Can you work these out from the model? Positions are in its coordinate system, mm. Face numbers are marked on the shaded views. A direction names the side the tool comes from. Round coordinates to 2 decimals unless told otherwise and drop trailing zeros. Order: outer loops, then holes, each group sorted by start corner. A loop starts at its lowest first (then second) coordinate and runs counter-clockwise, first axis right, second up. Notation, with made-up numbers: (76, 47) -> (84, 47) arc R14 cw to (84, 57) -> close; hole circle Ø10 at (20, -23.5). An arc over 180 degrees is marked (long way). One line per item, written item: value.
```python
from build123d import *

# Parameters (mm, degrees)
SKETCH1_R                = 6.35
BOSS_EXTRUDE1_DEPTH      = 19.05
SKETCH2_R                = 19.05
BOSS_EXTRUDE2_DEPTH      = 25.4
SKETCH3_R                = 25.4
BOSS_EXTRUDE3_DEPTH      = 38.1
SKETCH4_R                = 19.05
BOSS_EXTRUDE4_DEPTH      = 25.4
SKETCH6_R                = 6.35
BOSS_EXTRUDE5_DEPTH      = 28.194
SKETCH8_R                = 12.7
SKETCH8_R_2              = 9.525
BOSS_EXTRUDE7_DEPTH      = 38.1
BOSS_EXTRUDE8_DEPTH      = 1.5875
BOSS_EXTRUDE8_DEPTH_BACK = 1.5875
FILLET1_R                = 2.54
FILLET3_R                = 1.27
CUT_EXTRUDE1_REACH       = 145.927
SKETCH10_R               = 0.492787201


with BuildPart() as part:
    # Sketch1 → Boss-Extrude1 (new body)
    with BuildSketch(Plane(origin=(0, 0, 0), x_dir=(1, 0, 0), z_dir=(0, 1, 0))):
        with Locations(Location((0, 0, 0), (0, 0, 90))):
            Circle(SKETCH1_R)
    extrude(amount=BOSS_EXTRUDE1_DEPTH)

    # Sketch2 → Boss-Extrude2 (add)
    with BuildSketch(Plane(origin=(0, 19.05, 0), x_dir=(1, 0, 0), z_dir=(0, 1, 0))):
        with Locations(Location((0, 0, 0), (0, 0, 270))):
            Circle(SKETCH2_R)
    extrude(amount=BOSS_EXTRUDE2_DEPTH)

    # Sketch3 → Boss-Extrude3 (add)
    with BuildSketch(Plane(origin=(0, 44.45, 0), x_dir=(1, 0, 0), z_dir=(0, 1, 0))):
        with Locations(Location((0, 0, 0), (0, 0, 90))):
            Circle(SKETCH3_R)
    extrude(amount=BOSS_EXTRUDE3_DEPTH)

    # Sketch4 → Boss-Extrude4 (add)
    with BuildSketch(Plane(origin=(0, 82.55, 0), x_dir=(1, 0, 0), z_dir=(0, 1, 0))):
        with Locations(Location((0, 0, 0), (0, 0, 270))):
            Circle(SKETCH4_R)
    extrude(amount=BOSS_EXTRUDE4_DEPTH)

    # Sketch6 → Boss-Extrude5 (add)
    with BuildSketch(Plane(origin=(0, 107.95, 0), x_dir=(1, 0, 0), z_dir=(0, 1, 0))):
        with Locations(Location((0, 0, 0), (0, 0, 90))):
            Circle(SKETCH6_R)
    extrude(amount=BOSS_EXTRUDE5_DEPTH)

    # Sketch8 → Boss-Extrude7 (add)
    with BuildSketch(Plane(origin=(0, 0, 0), x_dir=(0, 0, -1), z_dir=(1, 0, 0))):
        with Locations(Location((0, 62.6872, 0), (0, 0, 180))):
            Circle(SKETCH8_R)
        with Locations(Location((0, 62.6872, 0), (0, 0, 180))):
            Circle(SKETCH8_R_2, mode=Mode.SUBTRACT)
    extrude(amount=BOSS_EXTRUDE7_DEPTH)

    # Sketch9 → Boss-Extrude8 (add, two sides: drawn at the far end of the back side and taken through both)
    with BuildSketch(Plane.XY.offset(-BOSS_EXTRUDE8_DEPTH_BACK)):
        with BuildLine():
            Line((8.114515419, 125.073963283), (6.806070155, 123.814961738))
            Line((6.806070155, 123.814961738), (-6.937623928, 123.814961738))
            ThreePointArc((-6.937623928, 123.814961738), (-7.582023221, 123.584458747), (-7.934028883, 122.997539593))
            Line((-7.934028883, 122.997539593), (-10.230756182, 111.473241157))
            ThreePointArc((-10.230756182, 111.473241157), (-10.582761844, 110.886322003), (-11.227161138, 110.655819012))
            Line((-11.227161138, 110.655819012), (-11.332644522, 110.655819012))
            ThreePointArc((-11.332644522, 110.655819012), (-12.11814153, 111.027419718), (-12.329049477, 111.870396866))
            Line((-12.329049477, 111.870396866), (-9.688493735, 125.119924761))
            ThreePointArc((-9.688493735, 125.119924761), (-9.336488073, 125.706843914), (-8.692088779, 125.937346906))
            Line((-8.692088779, 125.937346906), (6.085596345, 125.937346906))
            ThreePointArc((6.085596345, 125.937346906), (7.752909986, 127.03983771), (8.114515419, 125.073963283))
        make_face()
    extrude(amount=BOSS_EXTRUDE8_DEPTH + BOSS_EXTRUDE8_DEPTH_BACK)

    # Fillet1
    fillet1_edges = [part.edges().sort_by_distance(p)[0] for p in [
        (0, 82.55, 25.4),
        (0, 107.95, -19.05),
        (0, 19.05, -19.05),
        (0, 44.45, 25.4),
    ]]
    fillet(fillet1_edges, radius=FILLET1_R)

    # Fillet3
    fillet3_edges = [part.edges().sort_by_distance(p)[0] for p in [
        (0, 136.144, 6.35),
    ]]
    fillet(fillet3_edges, radius=FILLET3_R)

    # Sketch10 → Cut-Extrude1 (cut, up to next)
    with BuildSketch(Plane.XY.offset(1.5875), mode=Mode.PRIVATE) as cut_extrude1_sk1:
        with Locations((-11.315111441, 111.468988839)):
            Circle(SKETCH10_R)
    cut_extrude1_tool1 = extrude(cut_extrude1_sk1.sketch, amount=-CUT_EXTRUDE1_REACH, mode=Mode.PRIVATE) & part.part
    add(cut_extrude1_tool1.solids().sort_by_distance((-11.315111, 111.468989, 1.5875))[0], mode=Mode.SUBTRACT)


solid = part.part
```
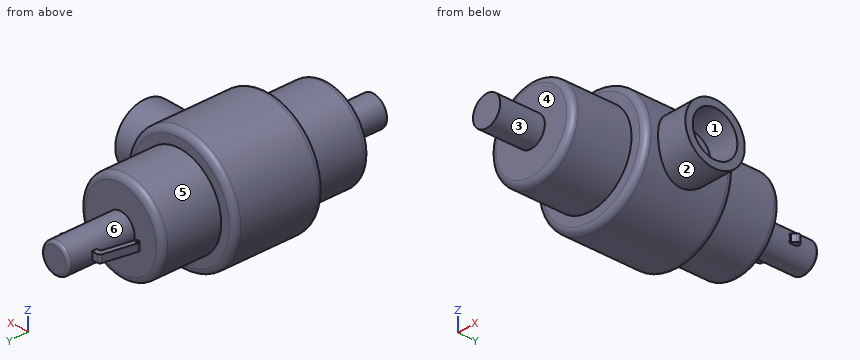
Q1. I want a section at C-C on x = 32. List the corners of the cut face in (y, z) for me (3 decimals), plus the area to 3 significant figures.
Answers below:
outline: circle Ø25.4 at (62.687, 0); hole circle Ø19.05 at (62.687, 0)
area: 222 mm^2
Q2. Please list where these lines run through material, in increasing order: line 1 along Y through (x, z) = (32, 0); line 2 along Y through (x, z) = (-6, -10.5); line 3 along Y through (x, z) = (29, 4).
Answers below:
line 1: 49.99 to 53.16, 72.21 to 75.39
line 2: 19.05 to 107.95
line 3: 50.63 to 54.04, 71.33 to 74.74
Q3. We'd pull the mould along Y, two halves only. Please class the marked faces 1, 2 and 3: released by +Y, released by -Y, zero draft, split by the parting line, or undercut.
Answers below:
face 1: undercut
face 2: split by the parting line
face 3: zero draft
Q4. On a 3-axis mill with a long thin cutter (end or side, diameter ignored), from which of +Z, -Z, +X, -X, +Y, -Y can I reach the whole of each face in a straight line? I mean the marked faces 4, 5 and 6. Say none if no direction works.
Answers below:
face 4: -Y
face 5: +Y
face 6: none
Q5. Will these pins go through, and if not, where does the flat tip stop? pin 1 Ø1.9 at (x, y) = (7.5, 125.5) entering from +Z; pin 2 Ø8 at (x, y) = (-17.5, 104) entering from -Z; pin 3 Ø12 at (x, y) = (12.5, 24) entering from -Z; pin 4 Ø0.5 at (x, z) = (6.5, 0) entering from -Y.
Answers below:
pin 1: z = 1.59
pin 2: z = -13.44
pin 3: z = -17.91
pin 4: y = 0
Q6. I want a section at B-B on y = 9. List the corners of the cut face in (x, z) for me.
Answers below:
outline: circle Ø12.7 at (0, 0)
Q7. I want a section at D-D on y = 103.5. List the corners of the cut face in (x, z) for me, plus the area to 3 significant figures.
Answers below:
outline: circle Ø38.1 at (0, 0)
area: 1,140 mm^2
